The model under review builds one solid part; all positions refer to its coordinate system, in mm. Coordinates: 2 decimals unless noted, no trailing zeros. Order: outer loops, then holes, each group sorted by start corner. A loop starts at its lowest first (then second) coordinate and runs counter-clockwise, first axis right, second up. Notation, with made-up numbers: (14.5, 42) -> (68.5, 42) arc R19 cw to (68.5, 56) -> close; hole circle Ø2 at (21.25, -34.75). An arc over 180 degrees is marked (long way). Use one line per item in the form item = value.
from build123d import *

# Parameters (mm, degrees)
SZKIC1_R                    = 3
DODANIE_WYCI_GNI_CIE2_DEPTH = 2.4
SZKIC2_R                    = 1.5
DODANIE_WYCI_GNI_CIE3_DEPTH = 35
ZAOKR_GLENIE2_R             = 1.2
WYTNIJ_WYCI_GNI_CIE1_DEPTH  = 1.94


with BuildPart() as part:
    # Szkic1 → Dodanie-wyciągnięcie2 (new body)
    with BuildSketch(Plane.XY):
        with Locations((-1.860516246, 2.732142857)):
            Circle(SZKIC1_R)
    extrude(amount=DODANIE_WYCI_GNI_CIE2_DEPTH)

    # Szkic2 → Dodanie-wyciągnięcie3 (add)
    with BuildSketch(Plane(origin=(0, 0, 0), x_dir=(-1, 0, 0), z_dir=(0, 0, -1))):
        with Locations((1.860516246, 2.732142857)):
            Circle(SZKIC2_R)
    extrude(amount=DODANIE_WYCI_GNI_CIE3_DEPTH)

    # Zaokrąglenie2
    zaokr_glenie2_edges = [part.edges().sort_by_distance(p)[0] for p in [
        (-4.860516246, 2.732142857, 2.4),
    ]]
    fillet(zaokr_glenie2_edges, radius=ZAOKR_GLENIE2_R)

    # Szkic3 → Wytnij-wyciągnięcie1 (cut)
    with BuildSketch(Plane.XY.offset(2.4)):
        with BuildLine():
            Line((-1.859548318, 2.959091853), (-0.575649693, 5.316481314))
            ThreePointArc((-0.575649693, 5.316481314), (-0.297886623, 5.158637444), (-0.039271083, 4.97106076))
            Line((-0.039271083, 4.97106076), (-1.329373025, 2.669425378))
            Line((-1.329373025, 2.669425378), (-0.183967515, 2.043621837))
            ThreePointArc((-0.183967515, 2.043621837), (-0.320475658, 1.776553075), (-0.499159616, 1.535654258))
            Line((-0.499159616, 1.535654258), (-1.621312108, 2.148584891))
            Line((-1.621312108, 2.148584891), (-2.819933608, 0.01015725))
            ThreePointArc((-2.819933608, 0.01015725), (-3.083174674, 0.117799023), (-3.33454353, 0.250826496))
            Line((-3.33454353, 0.250826496), (-2.145142944, 2.434706401))
            Line((-2.145142944, 2.434706401), (-3.258687897, 3.042935511))
            ThreePointArc((-3.258687897, 3.042935511), (-3.162842423, 3.328316127), (-3.009463836, 3.587359481))
            Line((-3.009463836, 3.587359481), (-1.859548318, 2.959091853))
        make_face()
    extrude(amount=-WYTNIJ_WYCI_GNI_CIE1_DEPTH, mode=Mode.SUBTRACT)


solid = part.part
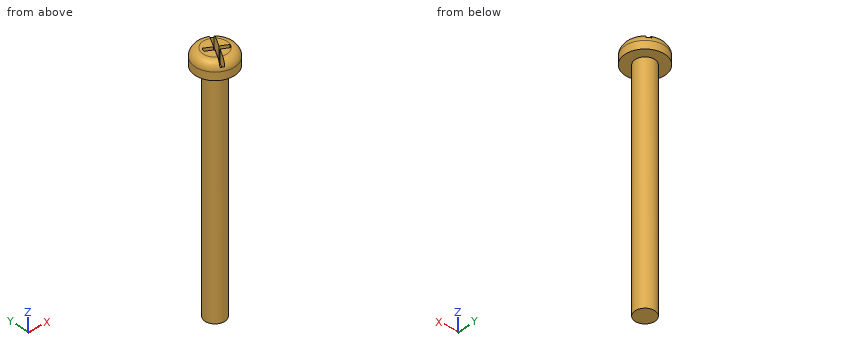
Item 1: Clearance check with flat-ended pins moving along their axes: pin 1 (1.5 mm diameter, centred on y = 1, z = -22, fed in from -X); pin 2 (1 mm diameter, centred on y = 4, z = -24, fed in from +X); pin 3 (1.5 mm diameter, centred on x = 0, z = -7.5, fed in from +Y). State where each tip first meets the part, or that it passes through.
Results found:
pin_1 = -2.99
pin_2 = -0.57
pin_3 = 3.74
Item 2: We need section A-A (z = -27). Write out the cut boundary in (x, y).
Results found:
outline = circle Ø3 at (-1.86, 2.73)
Item 3: To check wall thickness, follow L1, parallel to X at y = 1.5, z = 1; L2, parallel to X at y = 2.75, z = -9.5; L3, parallel to Z at x = -2.5, y = 3.25. State the ranges of each line that lie inside material, in increasing order. Write a range as from..to.
Results found:
L1 = -4.6..-2.65, -1.98..0.87
L2 = -3.36..-0.36
L3 = -35..0.46
